The model under review builds one solid part; all positions refer to its coordinate system, in mm. Give positions to 0.01 mm unless a question says otherwise; leave off trailing zeros. Write each loop counter-clockwise with the first axis right and the second up, starting at its lowest first coordinate (ties: lowest second). Pieces come first, ordered by that corner, then holes. Notation, with made-up numbers: M 6,53.25 L 53,53.25 A11 ccw 53,66.25 Z; hole C -25,21 d3. An arc over 180 degrees is marked long. Write item = value, one per line. Start each with the question number.
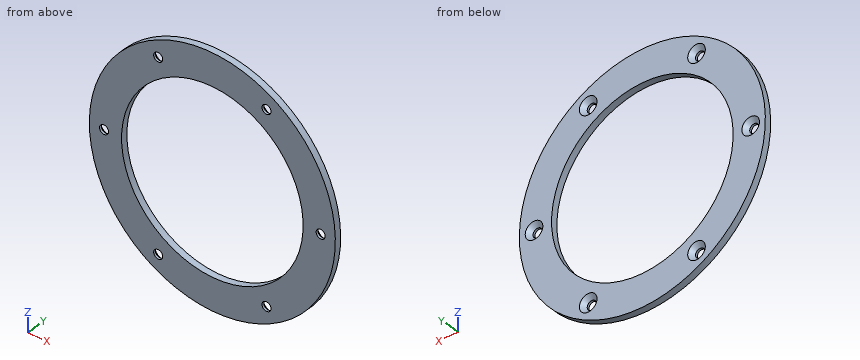
```python
from build123d import *

# Parameters (mm, degrees)
SKETCH_1_W          = 15
SKETCH_1_H          = 3
SKETCH_2_R          = 2.1
CUT_EXTRUDE_1_DEPTH = 10
CHAMFER_1_SIZE      = 2


with BuildPart() as part:
    # 草图1 → 旋转1 (revolve)
    with BuildSketch(Plane.XY, mode=Mode.PRIVATE) as revolve_1_sk:
        with Locations((49.78, 4.365902373)):
            Rectangle(SKETCH_1_W, SKETCH_1_H)
    revolve(revolve_1_sk.sketch.rotate(Axis((0, 0, 0), (0, 1, 0)), 90), axis=Axis((0, 0, 0), (0, 1, 0)))

    # 草图2 → 切除-拉伸1 (cut)
    with BuildSketch(Plane(origin=(0, 5.865902373, 0), x_dir=(1, 0, 0), z_dir=(0, 1, 0))):
        with Locations(Location((-50.45, 0, 0), (0, 0, 270))):
            Circle(SKETCH_2_R)
        with Locations(Location((-25.225, 43.690981621, 0), (0, 0, 270))):
            Circle(SKETCH_2_R)
        with Locations(Location((25.225, 43.690981621, 0), (0, 0, 270))):
            Circle(SKETCH_2_R)
        with Locations(Location((50.45, 0, 0), (0, 0, 270))):
            Circle(SKETCH_2_R)
        with Locations(Location((25.225, -43.690981621, 0), (0, 0, 270))):
            Circle(SKETCH_2_R)
        with Locations(Location((-25.225, -43.690981621, 0), (0, 0, 270))):
            Circle(SKETCH_2_R)
    extrude(amount=-CUT_EXTRUDE_1_DEPTH, mode=Mode.SUBTRACT)

    # 倒角1
    chamfer_1_edges = [part.edges().sort_by_distance(p)[0] for p in [
        (-50.45, 5.865902373, -2.1),
        (-25.225, 5.865902373, 41.590981621),
        (25.225, 5.865902373, 41.590981621),
        (50.45, 5.865902373, -2.1),
        (25.225, 5.865902373, -45.790981621),
        (-25.225, 5.865902373, -45.790981621),
    ]]
    chamfer(chamfer_1_edges, length=CHAMFER_1_SIZE)


solid = part.part
```
Item 1: We need section D-D, the plane y = 4.95. Write out the cut boundary in (x, z) (3 decimals).
Item 2: We need section A-A, the plane z = 0. Write out the cut boundary in (x, y).
Item 3: Clearance check with flat-ended pins moving along their axes: P1, Ø6.5, axis at x = -50.45, z = 0, coming from the +Y side; P2, Ø1, axis at y = 3.5, z = -29, coming from the +X side; P3, Ø5.5, axis at x = 50.45, z = 0, coming from the +Y side. State where each tip first meets the part, or that it passes through.
Item 4: We need section C-C, the plane z = -12.5. Write out the cut boundary in (x, y), and give its area (3 significant figures).
Item 5: We need section B-B, the plane x = 0. Write out the cut boundary in (y, z), and give its area (3 significant figures).
Item 6: To check wall thickness, follow probe 1 along X at (y, z) = (4.6, -1); probe 2 along X at (y, z) = (5.25, -45); probe 3 along Z at (x, y) = (-26.5, 5). State the ranges of each line that lie inside material, in increasing order. Write a range as [from, to].
Worked out:
q1.outline = C 0,0 d114.56; hole C -50.45,0 d6.368; hole C 0,0 d84.56; hole C -25.225,-43.691 d6.368; hole C -25.225,43.691 d6.368; hole C 25.225,-43.691 d6.368; hole C 25.225,43.691 d6.368; hole C 50.45,0 d6.368
q2.outline = M -57.28,2.87 L -52.55,2.87 L -52.55,3.87 L -54.55,5.87 L -57.28,5.87 Z; M -48.35,2.87 L -42.28,2.87 L -42.28,5.87 L -46.35,5.87 L -48.35,3.87 Z; M 42.28,2.87 L 48.35,2.87 L 48.35,3.87 L 46.35,5.87 L 42.28,5.87 Z; M 52.55,2.87 L 57.28,2.87 L 57.28,5.87 L 54.55,5.87 L 52.55,3.87 Z
q3.P1 = 5.02
q3.P2 = 49.69
q3.P3 = 4.52
q4.outline = M -55.9,2.87 L -40.39,2.87 L -40.39,5.87 L -55.9,5.87 Z; M 40.39,2.87 L 55.9,2.87 L 55.9,5.87 L 40.39,5.87 Z
q4.area = 93.1 mm²
q5.outline = M 2.87,-57.28 L 5.87,-57.28 L 5.87,-42.28 L 2.87,-42.28 Z; M 2.87,42.28 L 5.87,42.28 L 5.87,57.28 L 2.87,57.28 Z
q5.area = 90.0 mm²
q6.probe_1 = [-57.27, -53.1], [-47.8, -42.27], [42.27, 47.8], [53.1, 57.27]
q6.probe_2 = [-35.44, -28.45], [-22, 22], [28.45, 35.44]
q6.probe_3 = [-50.78, -46.66], [-40.72, -32.94], [32.94, 40.72], [46.66, 50.78]
